Could you check a few things on this drawing? It's one solid part, dimensions in mm from its lowest x, y, z. A direction names the side the tool comes from. Coordinates: 2 decimals unless noted, no trailing zeros. Write each loop counter-clockwise with the first axis right and the second up, starting at its lowest first coordinate (ties: lowest second). Pieces come first, ordered by that corner, then holes. Notation, with made-up numbers: (-8, 5) - (33, 5) arc R8 cw to (33, 15) - close; hole circle Ø8 at (83, -30). An arc over 180 degrees is marked (long way). Answer as a JSON object with one key per item and string values. Group by question number.
1) On a 3-axis mill with a long thin cutter (end or side, diameter ignored), from which of +Z, -Z, +X, -X, +Y, -Y can I reach the whole of each face in a straight line? I mean the marked faces 1 and 2. Say none if no direction works.
2) Please list where these lines run through material, in increasing order: line 1 along Y through (x, z) = (11.75, 12); line 2 along X through (y, z) = (22.25, 9.25); line 3 along Y through (x, z) = (1, 19.5).
3) We'd pull the mould along X, two halves only. Please class the marked faces 3, 4, 5 and 6: released by +X, released by -X, zero draft, split by the parting line, or undercut.
4) Will these pins go through, and if not, where does the flat tip stop? pin 1 Ø8 at (x, y) = (3, 19) entering from -Z; pin 2 Ø5 at (x, z) = (8, 13.5) entering from +Y; pin 3 Ø3 at (y, z) = (12, 12) entering from -X; pin 4 Ø6 at (x, z) = (1.5, 7.5) entering from -Y.
5) If we section it at A-A (y = 12): Write out the boundary of the cut face in (x, z).
6) If we section it at C-C (x = 10): Write out the boundary of the cut face in (y, z).
7) If we section it at D-D (y = 20): Write out the boundary of the cut face in (x, z), plus the area to 3 significant figures.
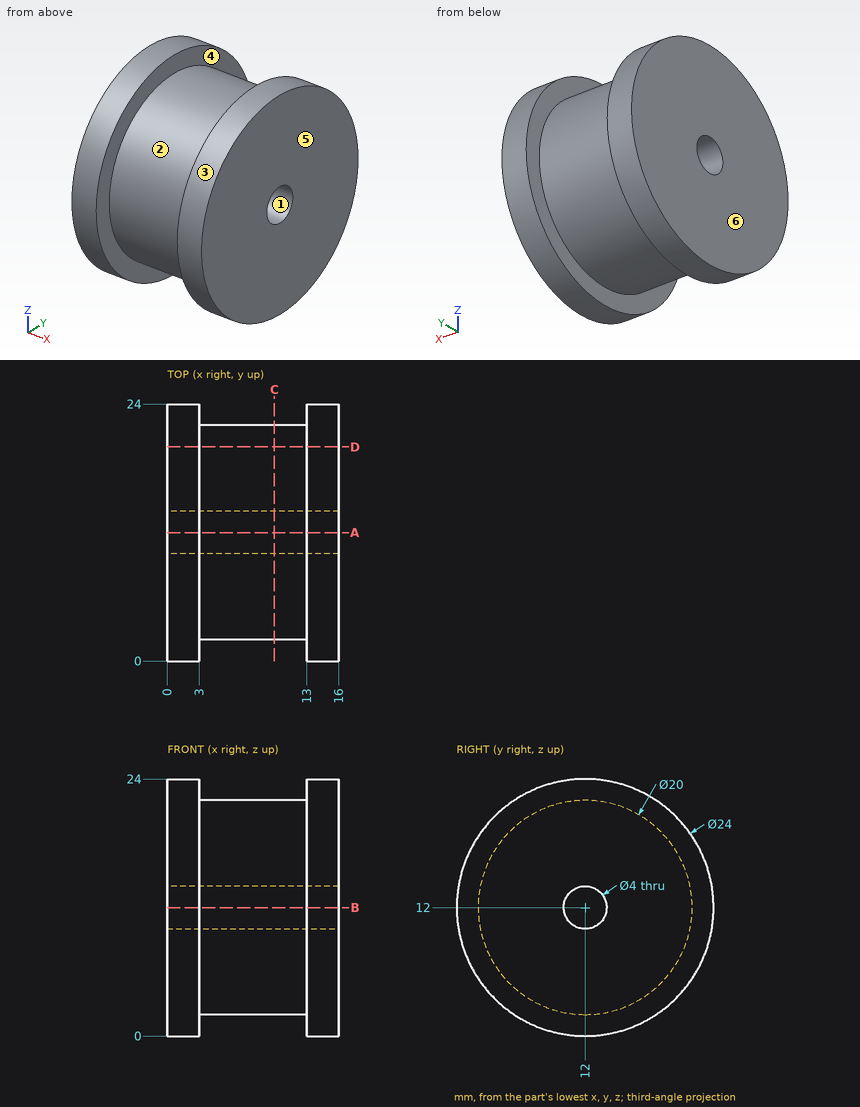
Here are the results:
{
 "1": {"face 1": "+X, -X", "face 2": "none"},
 "2": {"line 1": "y = 2 to 10, 14 to 22", "line 2": "x = 0 to 3, 13 to 16", "line 3": "y = 2.63 to 21.37"},
 "3": {"face 3": "zero draft", "face 4": "undercut", "face 5": "released by +X", "face 6": "released by -X"},
 "4": {"pin 1": "stops at z = 0.38", "pin 2": "stops at y = 22", "pin 3": "passes through", "pin 4": "stops at y = 0.09"},
 "5": {"outline": "(0, 0) - (3, 0) - (3, 2) - (13, 2) - (13, 0) - (16, 0) - (16, 10) - (0, 10) - close; (0, 14) - (16, 14) - (16, 24) - (13, 24) - (13, 22) - (3, 22) - (3, 24) - (0, 24) - close"},
 "6": {"outline": "circle Ø20 at (12, 12); hole circle Ø4 at (12, 12)"},
 "7": {"outline": "(0, 3.06) - (3, 3.06) - (3, 6) - (13, 6) - (13, 3.06) - (16, 3.06) - (16, 20.94) - (13, 20.94) - (13, 18) - (3, 18) - (3, 20.94) - (0, 20.94) - close", "area": "227 mm²"}
}
